```python
from build123d import *

# Parameters (mm, degrees)
F0_W     = 250
F0_H     = 160
F1_DEPTH = 25
F2_W     = 15
F2_H     = 15
F3_DEPTH = 25
F4_W     = 185
F4_H     = 100
F5_DEPTH = 25
F6_R     = 3
F7_DEPTH = 40
F8_R     = 3
F9_DEPTH = 40


with BuildPart() as f1:
    # F0 (on Top) → F1 (new body)
    with BuildSketch(Plane.XY):
        Rectangle(F0_W, F0_H)
    extrude(amount=F1_DEPTH)

    # F2 (on face) → F3 (cut)
    with BuildSketch(Plane.XY.offset(25)):
        with Locations((-117.5, 72.5)):
            Rectangle(F2_W, F2_H)
        with Locations((117.5, 72.5)):
            Rectangle(F2_W, F2_H)
        with Locations((117.5, -72.5)):
            Rectangle(F2_W, F2_H)
        with Locations((-117.5, -72.5)):
            Rectangle(F2_W, F2_H)
    extrude(amount=-F3_DEPTH, mode=Mode.SUBTRACT)

    # F4 (on face) → F5 (cut)
    with BuildSketch(Plane.XY.offset(25)):
        Rectangle(F4_W, F4_H)
    extrude(amount=-F5_DEPTH, mode=Mode.SUBTRACT)

    # F6 (on face) → F7 (cut)
    with BuildSketch(Plane.XZ.offset(80)):
        with Locations((0, 12.5)):
            Circle(F6_R)
    extrude(amount=-F7_DEPTH, mode=Mode.SUBTRACT)

    # F8 (on face) → F9 (cut)
    with BuildSketch(Plane(origin=(0, 80, 0), x_dir=(-1, 0, 0), z_dir=(0, 1, 0))):
        with Locations((0, 11.509229)):
            Circle(F8_R)
    extrude(amount=-F9_DEPTH, mode=Mode.SUBTRACT)


solid = f1.part
```
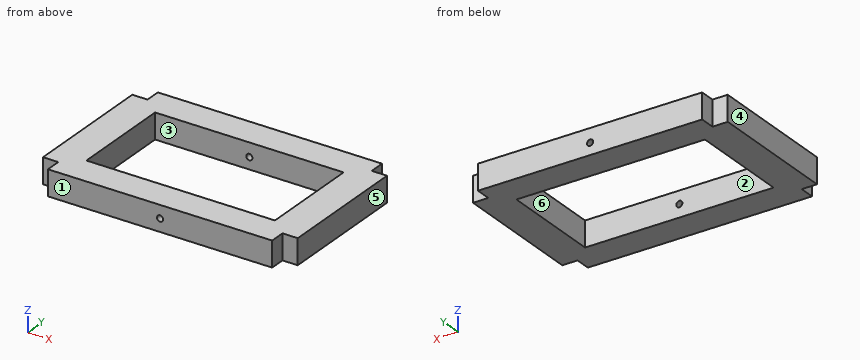
Here's how the part is built. I have some questions about the finished solid (model axes, mm). Face numbers are marked on the shaded views. A direction names the side the tool comes from. Coordinates: 2 decimals unless noted, no trailing zeros. Order: outer loops, then holes, each group sorted by start corner. A loop starts at its lowest first (then second) coordinate and runs counter-clockwise, first axis right, second up.
1) Imagine slicing it at B-B on y = -1. List the corners of the cut face in (x, z) for me, and give its area (4 significant figures).
2) Imagine slicing it at C-C on x = 63.5. List the corners of the cut face in (y, z) for me.
3) Which directions (+Z, -Z, +X, -X, +Y, -Y) give clear straight access to the entire face, cutting with the end or side of a thin tool? Please do the marked faces 5 and 6.
4) Will these pins go through, and if not, where does the flat tip stop? pin 1 (4.5 mm diameter, centred on y = -71.5, z = 12.5, fed in from +X); pin 2 (5 mm diameter, centred on x = 0, z = 12.5, fed in from -Y); pin 3 (7.5 mm diameter, centred on y = -76, z = 10, fed in from -X).
5) Imagine slicing it at A-A on x = 0. List the corners of the cut face in (y, z) for me.
6) I need wall thicknesses on line 1 (X direction, y = -1, z = 10.25); line 2 (Y direction, x = -38.5, z = 5.25); line 3 (Z direction, x = 0, y = 65.75). Which ranges of each line are inside material? Lowest first, please.
7) We'd pull the mould along X, two halves only. Please class the marked faces 1, 2, 3 and 4: +X half, -X half, draft (parallel to the pull), parting line (faces both ways), or undercut.
Response values:
1. outline: (-125, 0) - (-92.5, 0) - (-92.5, 25) - (-125, 25) - close; (92.5, 0) - (125, 0) - (125, 25) - (92.5, 25) - close
1. area: 1,625 mm2
2. outline: (-80, 0) - (-50, 0) - (-50, 25) - (-80, 25) - close; (50, 0) - (80, 0) - (80, 25) - (50, 25) - close
3. face 5: +Z, -Z, +X, +Y, -Y
3. face 6: +Z, -Z
4. pin 1: stops at x = 110
4. pin 2: stops at y = 50
4. pin 3: stops at x = -110
5. outline: (-80, 0) - (-50, 0) - (-50, 9.5) - (-80, 9.5) - close; (-80, 15.5) - (-50, 15.5) - (-50, 25) - (-80, 25) - close; (50, 0) - (80, 0) - (80, 8.51) - (50, 8.51) - close; (50, 14.51) - (80, 14.51) - (80, 25) - (50, 25) - close
6. line 1: x = -125 to -92.5, 92.5 to 125
6. line 2: y = -80 to -50, 50 to 80
6. line 3: z = 0 to 8.51, 14.51 to 25
7. face 1: draft
7. face 2: undercut
7. face 3: undercut
7. face 4: -X half
